Input: part model. Units: mm. Frame: model coordinates. A direction names the side the tool comes from. Round coordinates to 2 decimals unless told otherwise and drop trailing zeros. Loops run counter-clockwise (first coordinate to the right, second up) from the corner with the lowest first, then second, coordinate; pieces in that order, holes last. Notation, with made-up numbers: (72, 51) -> (106, 51) arc R13 ccw to (106, 58) -> close; hole circle Ø1 at (87.25, -29.5). An arc over 180 degrees is marked (long way). Answer as a JSON object with one key per item and string values. Group by question number.
Item 1: Section query A-A on y = 0. Return loops of the section in (x, z), and give its area (3 significant figures).
Item 2: Material intervals for line 1 (Y direction, x = 0, z = -3); line 2 (Y direction, x = 16.5, z = -6), sorted ascending. Write a range as [from, to].
Item 3: Section query D-D on x = 26. Return loops of the section in (y, z), and give its area (3 significant figures).
Item 4: Pin query (flat end, axial travel): pin 1 (1.5 mm diameter, centred on y = 20, z = -6, fed in from +X); pin 2 (1 mm diameter, centred on y = -18.5, z = -2, fed in from +X); pin 3 (3 mm diameter, centred on y = 12.5, z = -3.5, fed in from +X). Return the tip coordinate at first contact, or that it passes through.
Item 5: Draft query along Y for faces 3 (the conical face through (-0.805, -20.158, -0.826)), 4 (the flat face through (6.2, 20.4, 0)), 5 (the cylindrical face through (-29.97, 1.32, -4.93)). Return one class per face: released by +Y, released by -Y, zero draft, split by the parting line, or undercut.
Item 6: Section query C-C on z = -6.25. Return loops of the section in (x, y), and give its area (3 significant figures).
Item 7: Set-up query: faces 1 (the flat face through (6.2, 20.4, -10)), 2 (the flat face through (-6, 21, -5)). Return all of +Z, -Z, +X, -X, +Y, -Y with unobstructed straight access to the full face (end or side cutting, diameter ignored); none if empty.
Item 8: Section query B-B on x = 0. Return loops of the section in (y, z), and give its area (3 significant figures).
from build123d import *

# Parameters (mm, degrees)
SKETCH1_R           = 30
BOSS_EXTRUDE1_DEPTH = 10
CHAMFER1_SIZE       = 1


with BuildPart() as part:
    # Sketch1 → Boss-Extrude1 (new body)
    with BuildSketch(Plane.XY):
        Circle(SKETCH1_R)
        with BuildLine():
            ThreePointArc((-6, 19.078784028), (0, -20), (6, 19.078784028))
            Line((6, 19.078784028), (6, 22.078784028))
            Line((6, 22.078784028), (-6, 22.078784028))
            Line((-6, 22.078784028), (-6, 19.078784028))
        make_face(mode=Mode.SUBTRACT)
    extrude(amount=-BOSS_EXTRUDE1_DEPTH)

    # Chamfer1
    chamfer1_edges = [part.edges().sort_by_distance(p)[0] for p in [
        (0, -20, -10),
        (0, -20, 0),
    ]]
    chamfer(chamfer1_edges, length=CHAMFER1_SIZE)


solid = part.part
Solved:
{
 "1": {"outline": "(-30, -10) -> (-21, -10) -> (-20, -9) -> (-20, -1) -> (-21, 0) -> (-30, 0) -> close; (20, -9) -> (21, -10) -> (30, -10) -> (30, 0) -> (21, 0) -> (20, -1) -> close", "area": "198 mm²"},
 "2": {"line 1": "[-30, -20], [22.08, 30]", "line 2": "[-25.05, -11.3], [11.3, 25.05]"},
 "3": {"outline": "(-14.97, -10) -> (14.97, -10) -> (14.97, 0) -> (-14.97, 0) -> close", "area": "299 mm²"},
 "4": {"pin 1": "x = 23.01", "pin 2": "x = 24", "pin 3": "x = 27.91"},
 "5": {"face 3": "undercut", "face 4": "zero draft", "face 5": "split by the parting line"},
 "6": {"outline": "circle Ø60 at (0, 0); hole (-6, 19.08) arc R20 ccw (long way) to (6, 19.08) -> (6, 22.08) -> (-6, 22.08) -> close", "area": "1,540 mm²"},
 "7": {"face 1": "-Z, +X, -X, +Y, -Y", "face 2": "+Z, -Z"},
 "8": {"outline": "(-30, -10) -> (-21, -10) -> (-20, -9) -> (-20, -1) -> (-21, 0) -> (-30, 0) -> close; (22.08, -10) -> (30, -10) -> (30, 0) -> (22.08, 0) -> close", "area": "178 mm²"}
}
